```python
from build123d import *

# Parameters (mm, degrees)
F0_R     = 1.651
F1_DEPTH = 1.524


with BuildPart() as f1:
    # F0 (on Top) → F1 (new body)
    with BuildSketch(Plane.XY):
        with BuildLine():
            Line((-36.648669, -1.108164), (-3.175, -2.38125))
            ThreePointArc((-3.175, -2.38125), (3.96875, 0), (-3.175, 2.38125))
            Line((-3.175, 2.38125), (-36.648669, 1.108164))
            ThreePointArc((-36.648669, 1.108164), (-39.744666, 3.172706), (-42.674907, 0.878972))
            Line((-42.674907, 0.878972), (-65.786, 0))
            Line((-65.786, 0), (-42.674907, -0.878972))
            ThreePointArc((-42.674907, -0.878972), (-39.744666, -3.172706), (-36.648669, -1.108164))
        make_face()
        with Locations((-39.624, 0)):
            Circle(F0_R, mode=Mode.SUBTRACT)
        Circle(F0_R, mode=Mode.SUBTRACT)
    extrude(amount=F1_DEPTH)


solid = f1.part
```
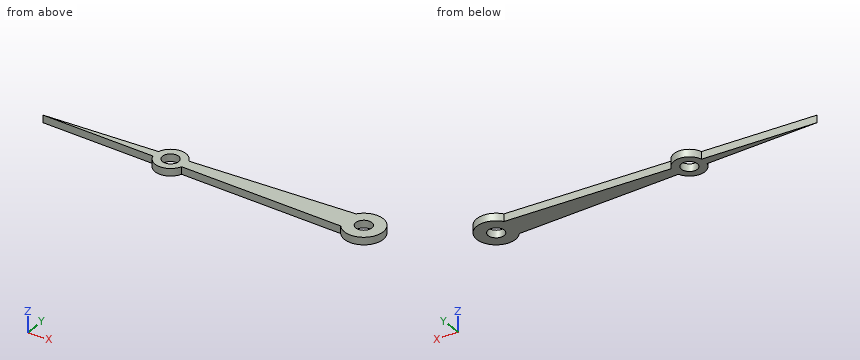
Geometry: final body of the model. Coordinates: model frame, mm. Give positions to 0.01 mm unless a question says otherwise; leave off trailing zeros. Order: outer loops, then holes, each group sorted by start corner. A loop starts at its lowest first (then second) coordinate and runs counter-clockwise, first axis right, second up. Notation, with made-up numbers: M -11,39.5 L 30,39.5 A31 cw 30,74.5 Z; hole C 33.25,11 d5. An arc over 180 degrees is marked long. Answer as CSV lines item,"result". Start each with the question number.
1) Cut plane C-C (x = -9). Output: boundary loops of the cut face in (y, z), then the cut area to 3 significant figures.
2) First-contact query: P1, Ø1, axis at x = -23, y = 2.5, coming from the +Z side. Flat tip, straight axial feed; report the tip coordinate or a pass-through.
3) Cut plane B-B (z = 1.05). State how many separate pieces and enclosed holes the cut face has, then the cut area to 3 significant figures.
4) Line query: line 1 (Y direction, x = 0, z = 0.9); line 2 (Y direction, x = -11, z = 0.9); line 3 (Y direction, x = -7.5, z = 0.8). Output: solid intervals per line, ascending. Write a range as from..to.
5) Cut plane A-A (x = 0). Output: boundary loops of the cut face in (y, z), then the cut area to 3 significant figures.
Findings below:
1,outline,"M -2.16,0 L 2.16,0 L 2.16,1.52 L -2.16,1.52 Z"
1,area,"6.58 mm²"
2,P1,"passes through"
3,separate pieces,"1"
3,enclosed holes,"2"
3,area,"198 mm²"
4,line 1,"y = -3.97..-1.65, 1.65..3.97"
4,line 2,"y = -2.08..2.08"
4,line 3,"y = -2.22..2.22"
5,outline,"M -3.97,0 L -1.65,0 L -1.65,1.52 L -3.97,1.52 Z; M 1.65,0 L 3.97,0 L 3.97,1.52 L 1.65,1.52 Z"
5,area,"7.06 mm²"
